Part print with two shaded views. Sizes in mm from the minimum x, y, z corner. A direction names the side the tool comes from. Give positions to 0.01 mm unless a question says otherwise; leave off trailing zeros. Order: outer loops, then holes, each group sorted by start corner. A loop starts at its lowest first (then second) coordinate and runs counter-clockwise, first axis right, second up. Notation, with made-up numbers: M 50,49 L 60,49 A17 ccw 60,61 Z; hole C 50.25,89.5 d3. An arc over 180 degrees is marked long. Return JSON: item names as keys, results as strings.
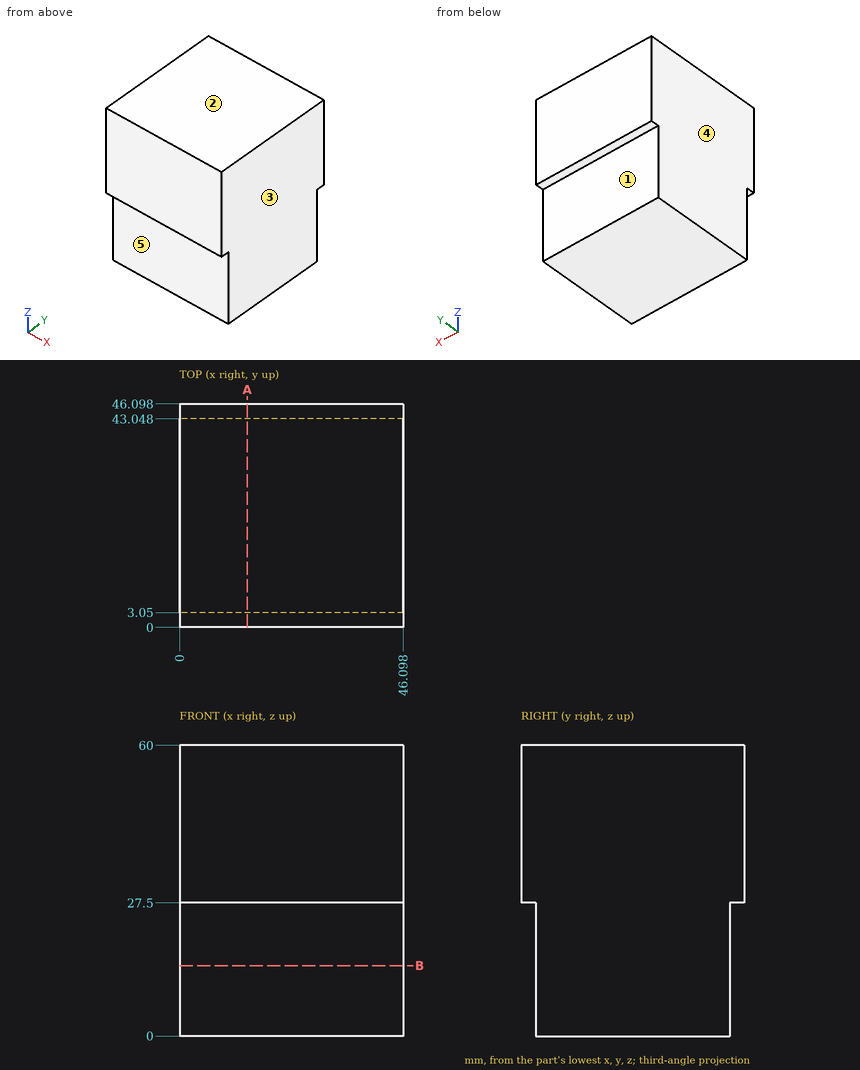
Q1. Two-plate mould, pull along X, no slides. Class the marked faces 3, 4 and 5: +X half, -X half, draft (parallel to the pull), parting line (faces both ways), or undercut.
Established:
{"face 3": "+X half", "face 4": "-X half", "face 5": "draft"}
Q2. Band-saw the part on A-A (x = 14). Give the cut face in (y, z), then the cut area to 3 significant figures.
Established:
{"outline": "M 0,27.5 L 3.05,27.5 L 3.05,0 L 43.05,0 L 43.05,27.5 L 46.1,27.5 L 46.1,60 L 0,60 Z", "area": "2,600 mm²"}
Q3. Probe line 1 along Y through (x, z) = (4, 12); line 2 along Z through (x, y) = (20, 44.5). List the from-to ranges inside material, lowest first.
Established:
{"line 1": "y = 3.05 to 43.05", "line 2": "z = 27.5 to 60"}
Q4. Band-saw the part on B-B (z = 14.5). Give the cut face in (x, y).
Established:
{"outline": "M 0,3.05 L 46.1,3.05 L 46.1,43.05 L 0,43.05 Z"}
Q5. Pin check, flat tips, straight feed: pin 1 (3 mm diameter, centred on x = 23.5, z = 49.5, fed in from -Y); pin 2 (14 mm diameter, centred on x = 19, z = 13, fed in from -Y); pin 3 (0.9 mm diameter, centred on x = 11.5, y = 44, fed in from -Z). Stop position of each tip, or through.
Established:
{"pin 1": "stops at y = 0", "pin 2": "stops at y = 3.05", "pin 3": "stops at z = 27.5"}
Q6. 3-axis set-ups, long thin cutter, end or side, ignore diameter. For the marked faces 1 and 2: which of +Z, -Z, +X, -X, +Y, -Y reach the whole face in a straight line?
Established:
{"face 1": "-Z, +X, -X, +Y", "face 2": "+Z, +X, -X, +Y, -Y"}
